from build123d import *

# Parameters (mm, degrees)
BASENUT_DEPTH = 16
DOMEFILLET_R  = 1


with BuildPart() as part:
    # BaseNutSke → BaseNut (new body)
    with BuildSketch(Plane(origin=(0, 0, 0), x_dir=(0, 0, -1), z_dir=(1, 0, 0))):
        Polygon((15, 8.660254038), (15, -8.660254038), (0, -17.320508076), (-15, -8.660254038), (-15, 8.660254038), (0, 17.320508076), align=None)
    extrude(amount=BASENUT_DEPTH)

    # DomeSke → Dome (revolve)
    with BuildSketch(Plane.XY, mode=Mode.PRIVATE) as dome_sk:
        with BuildLine():
            Line((34, 0), (0, 0))
            Line((0, 0), (0, 13.5))
            Line((0, 13.5), (20.5, 13.5))
            ThreePointArc((20.5, 13.5), (30.045941546, 9.545941546), (34, 0))
        make_face()
    revolve(dome_sk.sketch.rotate(Axis((0, 0, 0), (1, 0, 0)), 90), axis=Axis((0, 0, 0), (1, 0, 0)))

    # Sketch4 → DoubleChamfer (revolve, cut)
    with BuildSketch(Plane.XY):
        Polygon((0, 15), (2.783121635, 19.820508076), (13.216878365, 19.820508076), (16, 15), (18, 15), (18, 30), (-2, 30), (-2, 15), align=None)
    revolve(axis=Axis((0, 0, 0), (1, 0, 0)), mode=Mode.SUBTRACT)

    # TapDriSke → TapDrill (revolve, cut)
    with BuildSketch(Plane.XY, mode=Mode.PRIVATE) as tapdrill_sk:
        Polygon((0, 8.75), (27, 8.75), (32.257530416, 0), (0, 0), align=None)
    revolve(tapdrill_sk.sketch.rotate(Axis((0, 0, 0), (1, 0, 0)), 90), axis=Axis((0, 0, 0), (1, 0, 0)), mode=Mode.SUBTRACT)

    # EndChamferSketch → EndChamfer (revolve, cut)
    with BuildSketch(Plane.XY):
        Polygon((-0.0254, 10), (0.0254, 10), (0.988185365, 8.625), (-0.0254, 8.625), align=None)
    revolve(axis=Axis((0, 0, 0), (-1, 0, 0)), mode=Mode.SUBTRACT)

    # DomeFillet
    domefillet_edges = [part.edges().sort_by_distance(p)[0] for p in [
        (16, 0, -13.5),
    ]]
    fillet(domefillet_edges, radius=DOMEFILLET_R)


solid = part.part
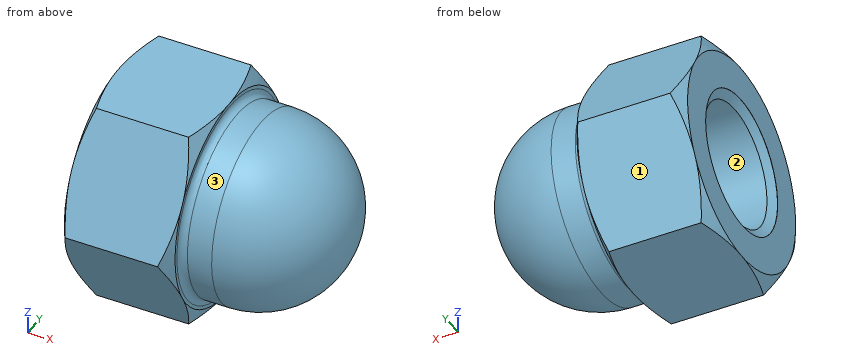
For this review, take the finished solid that the model builds, in its own axes (mm). Face numbers are marked on the shaded views. Give positions to 0.01 mm unless a question says otherwise; leave off trailing zeros. Loops run counter-clockwise (first coordinate to the right, second up) from the corner with the lowest first, then second, coordinate; pieces in that order, holes last. Notation, with made-up numbers: (2.5, 6) - (45.5, 6) arc R13 cw to (45.5, 29) - close; hole circle Ø1 at (34, 44.5). An arc over 180 degrees is marked (long way). Write each question's results on one line, items separated by ' | '.
(1) Take a section at B-B (x = 15.5). Give the boundary of the cut face in (y, z).
Conclusion:
outline: (-15.58, -3.02) - (-10.41, -11.98) arc R15.87 ccw to (-5.17, -15) - (5.17, -15) arc R15.87 ccw to (10.41, -11.98) - (15.58, -3.02) arc R15.87 ccw to (15.58, 3.02) - (10.41, 11.98) arc R15.87 ccw to (5.17, 15) - (-5.17, 15) arc R15.87 ccw to (-10.41, 11.98) - (-15.58, 3.02) arc R15.87 ccw to start; hole circle Ø17.5 at (0, 0)
(2) Take a section at A-A (x = 3). Give the boundary of the cut face in (y, z), then the cut area to 3 significant figures.
Conclusion:
outline: (-17.32, 0) - (-8.66, -15) - (8.66, -15) - (17.32, 0) - (8.66, 15) - (-8.66, 15) - close; hole circle Ø17.5 at (0, 0) | area: 539 mm^2
(3) For line 1 along Y through (x, z) = (8.75, 0); line 2 along Z through (x, y) = (18, -1); line 3 along Y through (x, z) = (14, -6.75), list the stretches that pass through material, from the lowest coordinate up.
Conclusion:
line 1: -17.32 to -8.75, 8.75 to 17.32 | line 2: -13.46 to -8.69, 8.69 to 13.46 | line 3: -13.42 to -5.57, 5.57 to 13.42
(4) Draft analysis for pull direction Z (two halves, no side actions). For the marked faces 1, 2 and 3, state which applies: +Z half, -Z half, draft (parallel to the pull), parting line (faces both ways), or undercut.
Conclusion:
face 1: -Z half | face 2: undercut | face 3: parting line
(5) Take a section at C-C (x = 25). Give the boundary of the cut face in (y, z), then the cut area to 3 significant figures.
Conclusion:
outline: circle Ø25.46 at (0, 0); hole circle Ø17.5 at (0, 0) | area: 268 mm^2
(6) For pin 1 Ø5 at (y, z) = (-13, -7) entering from +X; pin 2 Ø3 at (x, z) = (21.5, -7.5) entering from -Y; pin 3 Ø4 at (x, y) = (27, -12.5) entering from -Z, all flat-tipped, find the tip position at first contact; note any pin that passes through.
Conclusion:
pin 1: x = 26.14 | pin 2: y = -12.06 | pin 3: z = -6.01
